Check sheet for the drawn part. Datum: minimum x, y, z corner. Units: mm. Give positions to 0.01 mm unless a question says otherwise; leave off trailing zeros. Write each loop counter-clockwise with the first axis right and the second up, starting at its lowest first coordinate (ties: lowest second). Pieces come first, ordered by that corner, then holes.
(1) Cross-section at B-B (x = 25.25). Record the boundary of the cut face in (y, z), and give its area (3 significant figures).
(2) Cross-section at A-A (z = 35.75). Record the boundary of the cut face in (x, y), and give its area (3 significant figures).
(3) Cross-section at D-D (z = 45). Record the boundary of the cut face in (x, y) (1 decimal).
(4) Cross-section at C-C (y = 1.5). Count the separate pieces of the cut face and the enclosed holes in it, and give its area (4 significant figures).
(5) Thickness scan on line 1 along Z through (x, y) = (25.25, 0.15); line 2 along Z through (x, y) = (44.5, 2.65) (1 decimal); line 3 along X through (y, z) = (0.35, 35.75). Record the ranges inside material, lowest first.
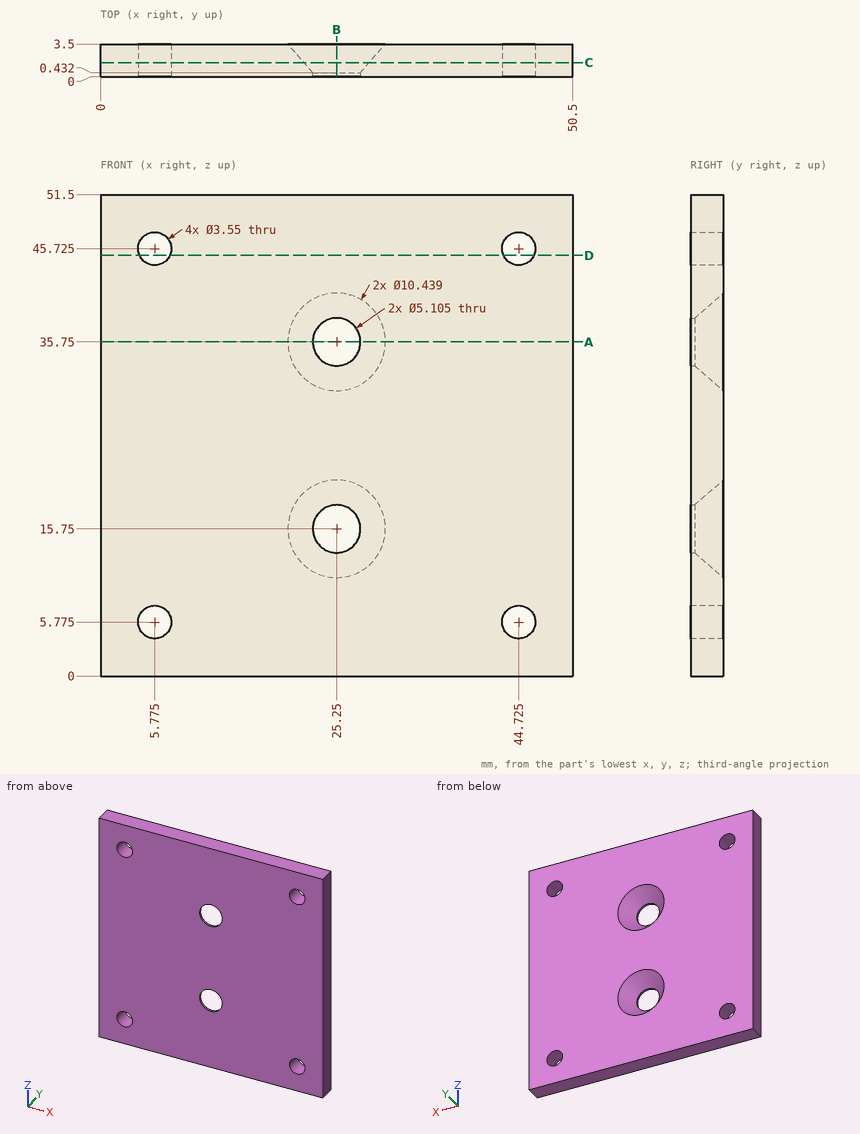
Reply:
1. outline: (0, 0) - (3.5, 0) - (3.5, 10.53) - (0.43, 13.2) - (0, 13.2) - close; (0, 18.3) - (0.43, 18.3) - (3.5, 20.97) - (3.5, 30.53) - (0.43, 33.2) - (0, 33.2) - close; (0, 38.3) - (0.43, 38.3) - (3.5, 40.97) - (3.5, 51.5) - (0, 51.5) - close
1. area: 128 mm2
2. outline: (0, 0) - (22.7, 0) - (22.7, 0.43) - (20.03, 3.5) - (0, 3.5) - close; (27.8, 0) - (50.5, 0) - (50.5, 3.5) - (30.47, 3.5) - (27.8, 0.43) - close
2. area: 151 mm2
3. outline: (0, 0) - (4.2, 0) - (4.2, 3.5) - (0, 3.5) - close; (7.4, 0) - (43.1, 0) - (43.1, 3.5) - (7.4, 3.5) - close; (46.3, 0) - (50.5, 0) - (50.5, 3.5) - (46.3, 3.5) - close
4. separate pieces: 1
4. enclosed holes: 6
4. area: 2,485 mm2
5. line 1: z = 0 to 13.2, 18.3 to 33.2, 38.3 to 51.5
5. line 2: z = 0 to 4, 7.5 to 44, 47.5 to 51.5
5. line 3: x = 0 to 22.7, 27.8 to 50.5
